CAD build for the part. Positions are in the model's coordinates, mm. Face numbers are marked on the shaded views. A direction names the side the tool comes from. Give positions to 0.01 mm unless a question says otherwise; leave off trailing zeros. Write each loop counter-clockwise with the first axis right and the second up, starting at its lowest first coordinate (ties: lowest second). Pieces come first, ordered by that corner, then holes. Notation, with made-up numbers: (38.25, 49) -> (64.25, 49) arc R28 cw to (64.25, 72) -> close; hole circle Ø9 at (50.25, 79). An arc over 180 degrees is marked (long way). Answer as a JSON object with one key per item and string values.
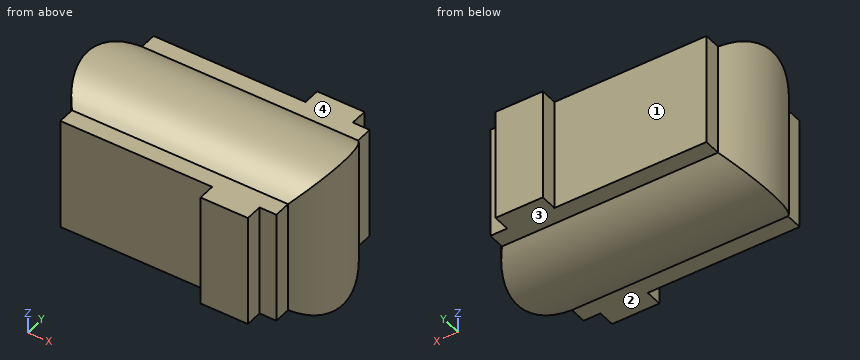
```python
from build123d import *

# Parameters (mm, degrees)
PAD_DEPTH    = 150
PAD001_DEPTH = 100


with BuildPart() as body:
    # Sketch → Pad (new body, symmetric)
    with BuildSketch(Plane.YZ):
        with BuildLine():
            ThreePointArc((30, 33.204857), (0, 44.75), (-30, 33.204857))
            Line((-30, 33.204857), (-50, 33.204857))
            Line((-50, 33.204857), (-50, -33.204857))
            Line((-50, -33.204857), (-30, -33.204857))
            ThreePointArc((-30, -33.204857), (0, -44.75), (30, -33.204857))
            Line((30, -33.204857), (50, -33.204857))
            Line((50, -33.204857), (50, 33.204857))
            Line((50, 33.204857), (30, 33.204857))
        make_face()
    extrude(amount=PAD_DEPTH, both=True)


with BuildPart() as body001:
    # Sketch001 → Pad001 (new body, symmetric)
    with BuildSketch(Plane.XY):
        with BuildLine():
            ThreePointArc((20, -30), (31.545143, 0), (20, 30))
            Line((20, 30), (20, 40))
            Line((20, 40), (10, 40))
            Line((10, 40), (10, 50))
            Line((10, 50), (-18, 50))
            Line((-18, 50), (-18, 40))
            Line((-18, 40), (-108, 40))
            Line((-108, 40), (-108, 30))
            ThreePointArc((-108, 30), (-119.545143, 0), (-108, -30))
            Line((-108, -30), (-108, -40))
            Line((-108, -40), (-18, -40))
            Line((-18, -40), (-18, -50))
            Line((-18, -50), (10, -50))
            Line((10, -50), (10, -40))
            Line((10, -40), (20, -40))
            Line((20, -40), (20, -30))
        make_face()
    extrude(amount=PAD001_DEPTH, both=True)

    # Boolean: intersect Body
    add(body.part, mode=Mode.INTERSECT)


solid = body001.part
```
1) Slice it at C-C (y = -12). List the corners of the cut face in (x, z).
Model answer:
{"outline": "(-117.91, -43.11) -> (29.91, -43.11) -> (29.91, 43.11) -> (-117.91, 43.11) -> close"}
2) 3-axis set-ups, long thin cutter, end or side, ignore diameter. For the marked faces 1, 2, 3 and 4: which of +Z, -Z, +X, -X, +Y, -Y reach the whole face in a straight line?
Model answer:
{"face 1": "+Z, -Z, -X, +Y", "face 2": "-Z, +X, -X, -Y", "face 3": "-Z, +X, -X, +Y", "face 4": "+Z, +X, -X, +Y"}
3) Slice it at D-D (y = 27.5). List the corners of the cut face in (x, z), then the cut area to 3 significant figures.
Model answer:
{"outline": "(-110.1, -35.3) -> (22.1, -35.3) -> (22.1, 35.3) -> (-110.1, 35.3) -> close", "area": "9,330 mm2"}
4) Wall check: probe 1 along Z at (x, y) = (-90.5, -1); probe 2 along Y at (x, z) = (-21.5, 15); probe 3 along Z at (x, y) = (-101.5, 30.5). Give the ranges that are in metal, low to high.
Model answer:
{"probe 1": "z = -44.74 to 44.74", "probe 2": "y = -40 to 40", "probe 3": "z = -33.2 to 33.2"}
5) Slice it at B-B (x = -70). List the corners of the cut face in (y, z).
Model answer:
{"outline": "(-40, -33.2) -> (-30, -33.2) arc R44.75 ccw to (30, -33.2) -> (40, -33.2) -> (40, 33.2) -> (30, 33.2) arc R44.75 ccw to (-30, 33.2) -> (-40, 33.2) -> close"}
6) Slice it at A-A (z = 29). List the corners of the cut face in (x, y), then the cut area to 3 significant figures.
Model answer:
{"outline": "(-108, -40) -> (-18, -40) -> (-18, -50) -> (10, -50) -> (10, -40) -> (20, -40) -> (20, -30) arc R44.75 ccw to (20, 30) -> (20, 40) -> (10, 40) -> (10, 50) -> (-18, 50) -> (-18, 40) -> (-108, 40) -> (-108, 30) arc R44.75 ccw to (-108, -30) -> close", "area": "11,800 mm2"}
7) Pin check, flat tips, straight feed: pin 1 (22 mm diameter, centred on x = -62.5, y = -44, fed in from +Z); pin 2 (8 mm diameter, centred on y = 46, z = -11, fed in from +X); pin 3 (1 mm diameter, centred on x = -68.5, z = -2, fed in from -Y). Stop position of each tip, or through.
Model answer:
{"pin 1": "stops at z = 33.2", "pin 2": "stops at x = 10", "pin 3": "stops at y = -40"}
